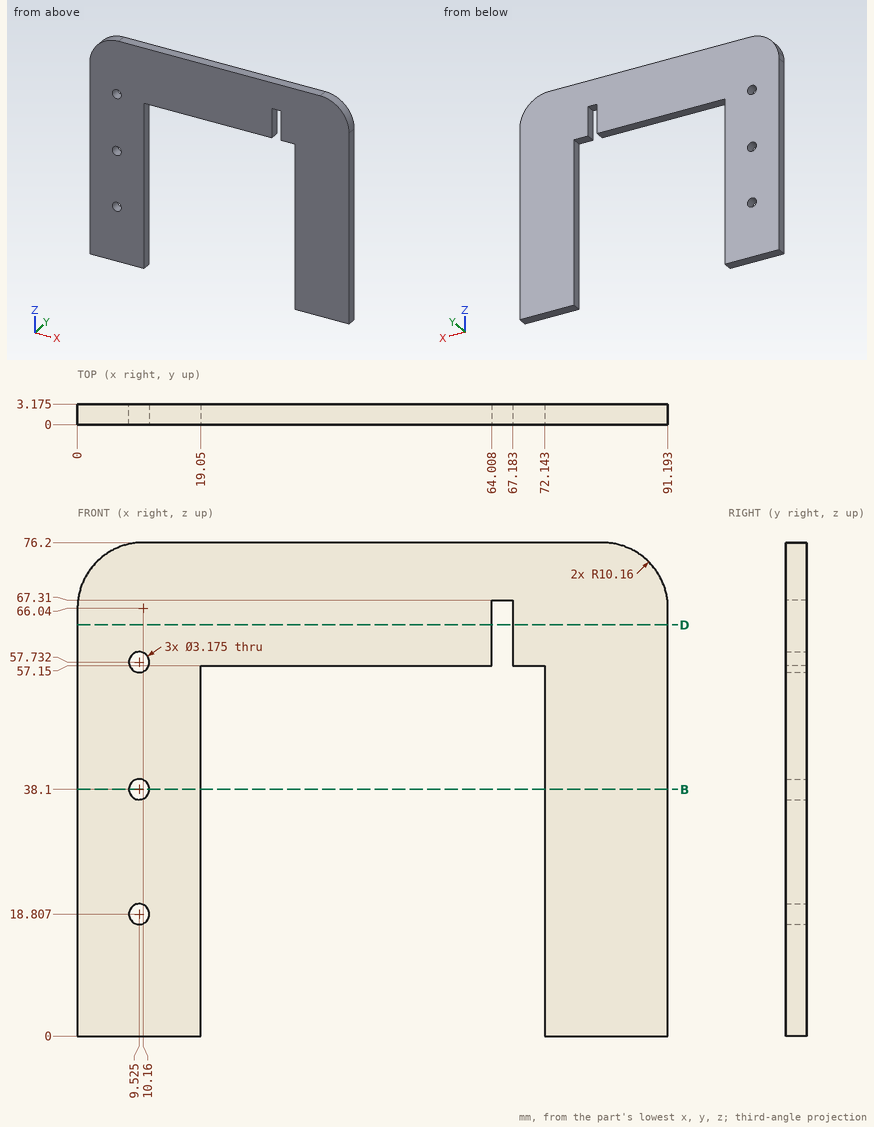
Geometry check sheet. Reference: drawing and pictorial views, mm from the part's lowest x, y, z. Round coordinates to 2 decimals unless told otherwise and drop trailing zeros. Order: outer loops, then holes, each group sorted by start corner. A loop starts at its lowest first (then second) coordinate and runs counter-clockwise, first axis right, second up.
Q1. Scan lines: L1, parallel to X at y = 1.2, z = 15.5; L2, parallel to X at y = 1.35, z = 18; L3, parallel to Z at x = 20.5, y = 2. Record each from-to range of solid material in increasing order.
Filled sheet:
L1: x = 0 to 19.05, 72.14 to 91.19
L2: x = 0 to 8.16, 10.89 to 19.05, 72.14 to 91.19
L3: z = 57.15 to 76.2
Q2. Cross-section at B-B, the plane z = 38.1. Give the number of separate pieces and of enclosed holes in the cut face, plus the area to 3 significant figures.
Filled sheet:
separate pieces: 3
enclosed holes: 0
area: 111 mm2
Q3. Cross-section at D-D, the plane z = 63.5. Enter the section's corners in (x, y) (1 decimal).
Filled sheet:
outline: (0, 0) - (64, 0) - (64, 3.2) - (0, 3.2) - close; (67.2, 0) - (91.2, 0) - (91.2, 3.2) - (67.2, 3.2) - close
Q4. Depth check by flat-ended pin: P1, Ø1.6, axis at x = 68.5, y = 1, coming from the -Z side; P2, Ø1.6, axis at x = 65, y = 2, coming from the -Z side. Enter the tip coordinate at first touch or a pass-through.
Filled sheet:
P1: stops at z = 57.15
P2: stops at z = 67.31
